Geometry check sheet. Reference: the model listing, model coordinates, mm. Give positions to 0.01 mm unless a question says otherwise; leave off trailing zeros. Write each loop counter-clockwise with the first axis right and the second up, starting at its lowest first coordinate (ties: lowest second). Pieces come first, ordered by that corner, then holes. Notation, with made-up numbers: (2, -3.75) -> (20, -3.75) arc R10 cw to (20, 0.25) -> close; hole circle Ø10 at (25, 34). An arc over 180 degrees is marked (long way). Write item = value, one per line. Start each with the question number.
1. Cross-section at B-B, the plane x = 0. Record the cut outline in (y, z).
2. Thickness scan on line 1 along X through (y, z) = (-25, 10.5); line 2 along Y through (x, z) = (0, 16); line 3 along X through (y, z) = (-29.5, 13). Record the ranges inside material, lowest first.
3. Cross-section at A-A, the plane y = -25. Record the cut outline in (x, z).
4. Mould release check, pull along X, two halves, no side actions. Record for faces 1 (the flat face through (-20, -25, 10)), 2 (the flat face through (9, -19, 19.912)), 3 (the cylindrical face through (9.54, -22, 13.83)): pulls with the +X half, pulls with the -X half, needs draft (parallel to the pull), parting line crosses it, or undercut.
5. Cross-section at C-C, the plane z = 13.75. Record the cut outline in (x, y), plus the area to 3 significant figures.
6. Cross-section at D-D, the plane y = -5. Record the cut outline in (x, z), plus the area to 3 significant figures.
7. Depth check by flat-ended pin: P1, Ø4, axis at x = 16, z = 16, coming from the +Y side; P2, Ø1, axis at x = 7.5, y = -13, coming from the -Z side. Enter the tip coordinate at first touch or a pass-through.
```python
from build123d import *

# Parameters (mm, degrees)
F0_W     = 40
F0_H     = 20
F1_DEPTH = 50
F2_R     = 25
F3_DEPTH = 50.001
F4_R     = 10
F5_DEPTH = 19.913378


with BuildPart() as f1:
    # F0 (on Front) → F1 (new body)
    with BuildSketch(Plane.XZ):
        with Locations((0, 9.912378)):
            Rectangle(F0_W, F0_H)
    extrude(amount=F1_DEPTH)

    # F2 (on Front) → F3 (cut, through all)
    with BuildSketch(Plane.XZ):
        with Locations((0, -15)):
            Circle(F2_R)
    extrude(amount=F3_DEPTH, mode=Mode.SUBTRACT)

    # F4 (on Top) → F5 (cut, through all)
    with BuildSketch(Plane.XY):
        with Locations((0, -25)):
            Circle(F4_R)
    extrude(amount=F5_DEPTH, mode=Mode.SUBTRACT)


solid = f1.part
```
Answers:
q1.outline = (-50, 10) -> (-35, 10) -> (-35, 19.91) -> (-50, 19.91) -> close; (-15, 10) -> (0, 10) -> (0, 19.91) -> (-15, 19.91) -> close
q2.line_1 = -20 to -10, 10 to 20
q2.line_2 = -50 to -35, -15 to 0
q2.line_3 = -20 to -8.93, 8.93 to 20
q3.outline = (-20, 0) arc R25 cw to (-10, 7.91) -> (-10, 19.91) -> (-20, 19.91) -> close; (10, 7.91) arc R25 cw to (20, 0) -> (20, 19.91) -> (10, 19.91) -> close
q4.face_1 = pulls with the -X half
q4.face_2 = needs draft
q4.face_3 = undercut
q5.outline = (-20, -50) -> (20, -50) -> (20, 0) -> (-20, 0) -> close; hole circle Ø20 at (0, -25)
q5.area = 1,690 mm^2
q6.outline = (-20, 0) arc R25 cw to (20, 0) -> (20, 19.91) -> (-20, 19.91) -> close
q6.area = 517 mm^2
q7.P1 = 0
q7.P2 = 8.69
